Autodesk Inventor part; units mm, degrees
ref_plane "Arbeitsebene1" through (0, 0, -66) normal (0, 0, 1) x (1, 0, 0)
ref_plane "YZ Plane" through (0, 0, 0) normal (1, 0, 0) x (0, 1, 0)
ref_plane "XZ Plane" through (0, 0, 0) normal (0, 1, 0) x (-1, 0, 0)
sketch "Skizze1" plane through (0, 0, 0) normal (0, 1, 0) x (-1, 0, 0)
  arc A0 (-19.7068, -62.5486) -> (19.7068, -62.5486) centre (0, 37) ccw
  line L0 (19.7068, -62.5486) -> (20, -64)
  arc A1 (-20, -64) -> (20, -64) centre (0, 35) ccw
  line L1 (-20, -64) -> (-19.7068, -62.5486)
  line L2 (0, -64.4804) -> (0, 0) construction
  point P0 (0, -64.4804)
  dimension "d0" = 2
  dimension "d1" = 101
  dimension "d2" = 40
  dimension "d3" = 35
extrude "Extrusion1" add sketch "Skizze1" along normal blind 100
ref_plane "Arbeitsebene1" through (0, 0, -66) normal (0, 0, 1) x (1, 0, 0)
sketch "Skizze2" plane through (0, 0, -66) normal (0, 0, 1) x (1, 0, 0)
  line L0 (20, 100) -> (-20, 100)
  point P0 (0, 0)
  point P1 (0, 78)
  point P2 (0, 50)
  point P3 (0, 22)
  dimension "d7" = 22
  dimension "d8" = 22
  dimension "d9" = 28
hole "Bohrung1" at (0, 78, -66) at (0, 50, -66) at (0, 22, -66) direction (0, 0, 1) diameter 4 end through all
sketch "Skizze3" plane through (0, 0, -66) normal (0, 0, 1) x (1, 0, 0)
  line L0 (-20, 0) -> (-20, 100)
  line L1 (-20, 89) -> (-15, 89)
  line L2 (-15, 89) -> (-15, 82)
  line L3 (-15, 82) -> (-20, 82)
  line L4 (20, 100) -> (-20, 100)
  line L5 (-20, 11) -> (-15, 11)
  line L6 (-15, 11) -> (-15, 18)
  line L7 (-15, 18) -> (-20, 18)
  line L8 (20, 0) -> (-20, 0)
  point P0 (0, 0)
  point P1 (-17.5, 82)
  point P2 (-17.5, 89)
  dimension "d17" = 5
  dimension "d18" = 7
  dimension "d19" = 11
  dimension "d20" = 5
  dimension "d21" = 7
  dimension "d22" = 11
extrude "Extrusion2" cut sketch "Skizze3" along normal through all
properties part number "214"
Part model, mm, in its own coordinate system. A direction names the side the tool comes from. Round coordinates to 2 decimals unless told otherwise and drop trailing zeros. Order: outer loops, then holes, each group sorted by start corner. A loop starts at its lowest first (then second) coordinate and runs counter-clockwise, first axis right, second up. Notation, with made-up numbers: M 29,6 L 57,6 A29 cw 57,28 Z; hole C -15,8 d8. An arc over 180 degrees is marked long. Put each result on its own line as item: value. Start each with the question number.
1. Drop flat-ended pins along their axis: pin 1 (6 mm diameter, centred on x = 8, y = 72.5, fed in from +Z); pin 2 (0.5 mm diameter, centred on y = 13, z = -64, fed in from -X). Give the stop position or say it passes through.
2. Slice it at B-B on y = 22.5. List the corners of the cut face in (x, z), then the cut area to 3 significant figures.
3. Slice it at A-A on x = 0. List the corners of the cut face in (y, z).
4. Drill centre lines: probe 1 along Y at (x, z) = (0, -65.15); probe 2 along Z at (x, y) = (-6.5, 39.5); probe 3 along Z at (x, y) = (10, 42.5). Where is each one in solid material? Low to high. Write a range as [from, to].
5. Slice it at D-D on x = 14. List the corners of the cut face in (y, z) (3 decimals).
6. Two-plate mould, pull along X, no slides. Class faces 1 (the face through (4.191, 49.3, -65.913)), 2 (the face through (1.2, 20.4, -65.2)), 3 (the face through (0, 0, -65)): +X half, -X half, draft (parallel to the pull), parting line (faces both ways), or undercut.
7. Tool access for faces 4 (the face through (-17, 82, -64)), 5 (the face through (-0.601, 79.908, -65.22)): list every direction of +Z, -Z, +X, -X, +Y, -Y with a clear straight run to the whole face (end or side of a thin tool).
8. Slice it at C-C on y = 78. List the corners of the cut face in (x, z), then the cut area to 3 significant figures.
Findings:
1. pin 1: z = -63.88
1. pin 2: x = -15
2. outline: M -20,-64 A101 ccw -1.94,-65.98 L -1.94,-64.46 A101.48 cw -19.71,-62.55 Z; M 1.94,-65.98 A101 ccw 20,-64 L 19.71,-62.55 A101.48 cw 1.94,-64.46 Z
2. area: 54.3 mm2
3. outline: M 0,-66 L 20,-66 L 20,-64.48 L 0,-64.48 Z; M 24,-66 L 48,-66 L 48,-64.48 L 24,-64.48 Z; M 52,-66 L 76,-66 L 76,-64.48 L 52,-64.48 Z; M 80,-66 L 100,-66 L 100,-64.48 L 80,-64.48 Z
4. probe 1: [0, 20], [24, 48], [52, 76], [80, 100]
4. probe 2: [-65.79, -64.27]
4. probe 3: [-65.5, -63.99]
5. outline: M 0,-65.025 L 100,-65.025 L 100,-63.51 L 0,-63.51 Z
6. face 1: parting line
6. face 2: undercut
6. face 3: draft
7. face 4: +Z, -Z, -X
7. face 5: +Z, -Z
8. outline: M -20,-64 A101 ccw -2,-65.98 L -2,-64.46 A101.48 cw -19.71,-62.55 Z; M 2,-65.98 A101 ccw 20,-64 L 19.71,-62.55 A101.48 cw 2,-64.46 Z
8. area: 54.1 mm2
